```python
from build123d import *

# Parameters (mm, degrees)
SKETCH1_W           = 180
SKETCH1_H           = 50
EXTRUDE1_DEPTH      = 200
SKETCH2_W           = 6
SKETCH2_H           = 50
EXTRUDE2_DEPTH      = 50
EXTRUDE3_DEPTH      = 477
EXTRUDE3_DEPTH_BACK = 40
SKETCH3_R           = 4
FILLET1_R           = 20


with BuildPart() as part:
    # Sketch1 → Extrude1 (new body)
    with BuildSketch(Plane(origin=(0, 0, 0), x_dir=(1, 0, 0), z_dir=(0, 1, 0))):
        Rectangle(SKETCH1_W, SKETCH1_H)
    extrude(amount=EXTRUDE1_DEPTH)

    # Sketch2 → Extrude2 (add)
    with BuildSketch(Plane.XZ):
        with Locations((-87, 0)):
            Rectangle(SKETCH2_W, SKETCH2_H)
        with Locations((87, 0)):
            Rectangle(SKETCH2_W, SKETCH2_H)
    extrude(amount=EXTRUDE2_DEPTH)

    # Sketch3 → Extrude3 (cut, two sides: drawn at the far end of the back side and taken through both)
    with BuildSketch(Plane.ZY.offset(-84).offset(-EXTRUDE3_DEPTH_BACK)):
        with Locations(Location((0, -25, 0), (0, 0, 180))):
            Circle(SKETCH3_R)
    extrude(amount=EXTRUDE3_DEPTH + EXTRUDE3_DEPTH_BACK, mode=Mode.SUBTRACT)

    # Fillet1
    fillet1_edges = [part.edges().sort_by_distance(p)[0] for p in [
        (-87, -50, -25),
        (-87, -50, 25),
        (87, -50, 25),
        (87, -50, -25),
    ]]
    fillet(fillet1_edges, radius=FILLET1_R)


solid = part.part
```
Geometry check sheet. Reference: the model listing, model coordinates, mm. A direction names the side the tool comes from. Give positions to 0.01 mm unless a question says otherwise; leave off trailing zeros. Loops run counter-clockwise (first coordinate to the right, second up) from the corner with the lowest first, then second, coordinate; pieces in that order, holes last. Notation, with made-up numbers: M 16.25,63 L 73.25,63 A25 ccw 73.25,88 Z; hole C 26,16.5 d1. An arc over 180 degrees is marked long. Write item = value, one per line.
(1) Sectioned sample at B-B, the plane z = 0. Record the cut outline in (x, y).
Answer below:
outline = M -90,-50 L -84,-50 L -84,-29 L -90,-29 Z; M -90,-21 L -84,-21 L -84,0 L 84,0 L 84,-21 L 90,-21 L 90,200 L -90,200 Z; M 84,-50 L 90,-50 L 90,-29 L 84,-29 Z
(2) Sectioned sample at A-A, the plane y = -25. Record the cut outline in (x, z).
Answer below:
outline = M -90,-25 L -84,-25 L -84,-4 L -90,-4 Z; M -90,4 L -84,4 L -84,25 L -90,25 Z; M 84,-25 L 90,-25 L 90,-4 L 84,-4 Z; M 84,4 L 90,4 L 90,25 L 84,25 Z
(3) Gauge pin test, flat ends, axial feed: pin 1 Ø15 at (x, z) = (26, 10) entering from -Y; pin 2 Ø10 at (x, y) = (-71.5, -7.5) entering from -Z. Record the tip position at first contact, or that the pin passes through.
Answer below:
pin_1 = 0
pin_2 = through
(4) Material ranges on line 1 (Y direction, x = -88.2, z = 0); line 2 (Y direction, x = -30, z = 18.5), recorded low to high. Write a range as [from, to].
Answer below:
line_1 = [-50, -29], [-21, 200]
line_2 = [0, 200]
(5) Release check for a two-part mould opening along Z. For faces 3 (the face through (84, -19, 0)), 4 (the face through (-1, 87, -25)), 5 (the face through (-86.958, -28.966, 0.521)) record: released by +Z, released by -Z, zero draft, split by the parting line, or undercut.
Answer below:
face_3 = zero draft
face_4 = released by -Z
face_5 = undercut
(6) Tool access check on faces 1 (the face through (-1, 87, 25)), 2 (the face through (-1, 0, 0)). Record the directions out of +Z, -Z, +X, -X, +Y, -Y that give a thin tool (end or side, any length) a straight path to the whole face; none if there is none.
Answer below:
face_1 = +Z, +X, -X, +Y, -Y
face_2 = +Z, -Z, -Y
(7) Sectioned sample at C-C, the plane x = -53. Record the cut outline in (y, z).
Answer below:
outline = M 0,-25 L 200,-25 L 200,25 L 0,25 Z
(8) Sectioned sample at D-D, the plane z = -16. Record the cut outline in (x, y).
Answer below:
outline = M -90,-46.7 L -84,-46.7 L -84,0 L 84,0 L 84,-46.7 L 90,-46.7 L 90,200 L -90,200 Z
